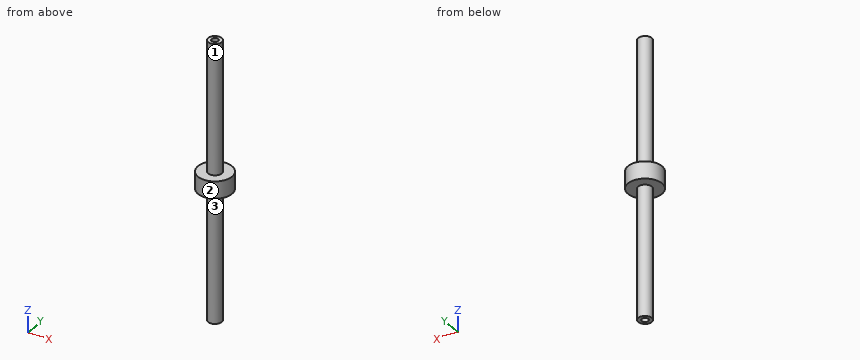
from build123d import *

# Parameters (mm, degrees)
SKETCH1_R               = 2
BOSS_EXTRUDE1_DEPTH     = 38
SKETCH2_R               = 5
BOSS_EXTRUDE2_DEPTH     = 5
SKETCH3_R               = 2
BOSS_EXTRUDE3_DEPTH     = 38
SKETCH4_R               = 1
CUT_EXTRUDE1_DEPTH      = 5
CUT_EXTRUDE2_DEPTH      = 82.308056181
CUT_EXTRUDE2_DEPTH_BACK = 5
SKETCH5_R               = 1


with BuildPart() as part:
    # Sketch1 → Boss-Extrude1 (new body)
    with BuildSketch(Plane.XY):
        Circle(SKETCH1_R)
    extrude(amount=BOSS_EXTRUDE1_DEPTH)

    # Sketch2 → Boss-Extrude2 (add)
    with BuildSketch(Plane.XY.offset(38)):
        Circle(SKETCH2_R)
    extrude(amount=BOSS_EXTRUDE2_DEPTH)

    # Sketch3 → Boss-Extrude3 (add)
    with BuildSketch(Plane.XY.offset(43)):
        Circle(SKETCH3_R)
    extrude(amount=BOSS_EXTRUDE3_DEPTH)

    # Sketch4 → Cut-Extrude1 (cut)
    with BuildSketch(Plane(origin=(0, 0, 0), x_dir=(-1, 0, 0), z_dir=(0, 0, -1))):
        Circle(SKETCH4_R)
    extrude(amount=-CUT_EXTRUDE1_DEPTH, mode=Mode.SUBTRACT)

    # Sketch5 → Cut-Extrude2 (cut, two sides: drawn at the far end of the back side and taken through both)
    with BuildSketch(Plane.XY.offset(81).offset(-CUT_EXTRUDE2_DEPTH_BACK)):
        with Locations(Location((0, 0, 0), (0, 0, 180))):
            Circle(SKETCH5_R)
    extrude(amount=CUT_EXTRUDE2_DEPTH + CUT_EXTRUDE2_DEPTH_BACK, mode=Mode.SUBTRACT)


solid = part.part
Could you check a few things on this model? Use its own coordinates, in mm. Face numbers are marked on the shaded views. A direction names the side the tool comes from. Round coordinates to 2 decimals unless told otherwise and drop trailing zeros. Loops run counter-clockwise (first coordinate to the right, second up) from the corner with the lowest first, then second, coordinate; pieces in that order, holes last. Notation, with made-up numbers: (53.25, -25.75) -> (74.25, -25.75) arc R31 cw to (74.25, 1.25) -> close; hole circle Ø1 at (14, 30.25). An arc over 180 degrees is marked (long way). Use CSV: the item, a comma, the result in double quotes.
(1) If I drill on probe 1 along Y at (x, z) = (0, 77.6); probe 2 along Z at (x, y) = (-0.25, 3.75); probe 3 along Y at (x, z) = (-0.75, 13), over which ranges is the centre line in solid material (lowest first)? Write a range as [from, to].
Return value:
probe 1,"y = [-2, -1], [1, 2]"
probe 2,"z = [38, 43]"
probe 3,"y = [-1.85, 1.85]"
(2) Suppose I cut it at C-C on z = 72. Write out the boundary of the cut face in (x, y).
Return value:
outline,"circle Ø4 at (0, 0)"
(3) Suppose I cut it at A-A on x = 0. Write out the boundary of the cut face in (y, z), plus the area to 3 significant figures.
Return value:
outline,"(-5, 38) -> (-2, 38) -> (-2, 0) -> (-1, 0) -> (-1, 5) -> (1, 5) -> (1, 0) -> (2, 0) -> (2, 38) -> (5, 38) -> (5, 43) -> (2, 43) -> (2, 81) -> (1, 81) -> (1, 76) -> (-1, 76) -> (-1, 81) -> (-2, 81) -> (-2, 43) -> (-5, 43) -> close"
area,"334 mm²"
(4) Will these pins go through, and if not, where does the flat tip stop? pin 1 Ø2 at (y, z) = (-0.5, 51) entering from -X; pin 2 Ø6 at (x, z) = (0.5, 24) entering from -Y; pin 3 Ø1.6 at (x, y) = (0, 0) entering from -Z.
Return value:
pin 1,"stops at x = -2"
pin 2,"stops at y = -2"
pin 3,"stops at z = 5"
(5) Suppose I cut it at D-D on x = 3. Write out the boundary of the cut face in (y, z).
Return value:
outline,"(-4, 38) -> (4, 38) -> (4, 43) -> (-4, 43) -> close"
(6) For the marked faces 1, 2 and 3, which set-ups out of +Z, -Z, +X, -X, +Y, -Y let a thin tool reach every point of the face, with its end or its side?
Return value:
face 1,"+Z"
face 2,"+Z, -Z"
face 3,"-Z"
